Read the model definition and answer for the solid it produces. Units are mm, in the model's axes. Face numbers are marked on the shaded views. Give positions to 0.01 mm unless a question says otherwise; leave off trailing zeros. Loops run counter-clockwise (first coordinate to the right, second up) from the corner with the lowest first, then second, coordinate; pieces in that order, holes last.
(1) Find section C-C, the plane y = -8.5. Write down the section's boundary in (x, z), then the cut area to 3 significant figures.
(2) Straight lines are drawn through the part: probe 1 along Y at (x, z) = (-1.75, -4.5); probe 2 along Z at (x, y) = (0.5, 0); probe 3 along X at (y, z) = (10, -0.25). For each, find the intervals that lie inside material, in ascending order.
(3) Find section B-B, the plane x = 0. Write down the section's boundary in (y, z).
(4) Each of these flat-tipped pins is pushed along its axis until it touches: P1, Ø1.5, axis at x = 3, y = 0, coming from the +Z side; P2, Ø4, axis at y = 3.5, z = -3.5, coming from the -X side. Where does it stop, or does it pass through?
(5) Find section A-A, the plane z = 0. Write down the section's boundary in (x, y), then the cut area to 3 significant figures.
(6) Determine the mould class of the marked faces 1, 2 and 3 for opening direction Y: pulls with the +Y half, pulls with the -Y half, needs draft (parallel to the pull), parting line crosses it, or undercut.
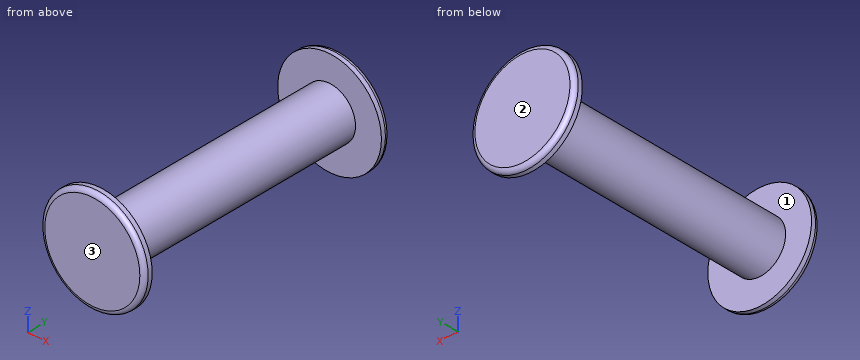
```python
from build123d import *

# Parameters (mm, degrees)
SKETCH_1_R             = 3
EXTRUDE_1_DEPTH        = 14.3
SKETCH_2_R             = 6
EXTRUDE_2_DEPTH        = 1
FILLET_1_R             = 0.5
FILLET_1_OF_MIRROR_1_R = 0.5


with BuildPart() as part:
    # 草图1 → 凸台-拉伸1 (new body, symmetric)
    with BuildSketch(Plane(origin=(0, 0, 0), x_dir=(1, 0, 0), z_dir=(0, 1, 0))):
        Circle(SKETCH_1_R)
    extrude(amount=EXTRUDE_1_DEPTH, both=True)

    # 草图2 → 凸台-拉伸2 (add)
    with BuildSketch(Plane(origin=(0, 14.3, 0), x_dir=(1, 0, 0), z_dir=(0, 1, 0))):
        Circle(SKETCH_2_R)
    extrude_2 = extrude(amount=EXTRUDE_2_DEPTH)

    # 圆角1
    fillet_1_edges = [part.edges().sort_by_distance(p)[0] for p in [
        (-6, 15.3, 0),
    ]]
    fillet(fillet_1_edges, radius=FILLET_1_R)

    # 镜向1: 凸台-拉伸2 across plane
    add(extrude_2.mirror(Plane.ZX))

    # 圆角1 of 镜向1
    fillet_1_of_mirror_1_edges = [part.edges().sort_by_distance(p)[0] for p in [
        (-6, -15.3, 0),
    ]]
    fillet(fillet_1_of_mirror_1_edges, radius=FILLET_1_OF_MIRROR_1_R)


solid = part.part
```
Entries:
1. outline: circle Ø6 at (0, 0)
1. area: 28.3 mm2
2. probe 1: y = -15.3 to -14.3, 14.3 to 15.3
2. probe 2: z = -2.96 to 2.96
2. probe 3: x = -2.99 to 2.99
3. outline: (-15.3, -5.5) arc R0.5 ccw to (-14.8, -6) - (-14.3, -6) - (-14.3, -3) - (14.3, -3) - (14.3, -6) - (14.8, -6) arc R0.5 ccw to (15.3, -5.5) - (15.3, 5.5) arc R0.5 ccw to (14.8, 6) - (14.3, 6) - (14.3, 3) - (-14.3, 3) - (-14.3, 6) - (-14.8, 6) arc R0.5 ccw to (-15.3, 5.5) - close
4. P1: stops at z = 1.98
4. P2: stops at x = -2.6
5. outline: (-6, -14.8) arc R0.5 ccw to (-5.5, -15.3) - (5.5, -15.3) arc R0.5 ccw to (6, -14.8) - (6, -14.3) - (3, -14.3) - (3, 14.3) - (6, 14.3) - (6, 14.8) arc R0.5 ccw to (5.5, 15.3) - (-5.5, 15.3) arc R0.5 ccw to (-6, 14.8) - (-6, 14.3) - (-3, 14.3) - (-3, -14.3) - (-6, -14.3) - close
5. area: 195 mm2
6. face 1: undercut
6. face 2: pulls with the +Y half
6. face 3: pulls with the -Y half
